Could you check a few things on this model? Use its own coordinates, in mm. A direction names the side the tool comes from. Coordinates: 2 decimals unless noted, no trailing zeros. Order: outer loops, then holes, each group sorted by start corner. A loop starts at its lowest first (then second) coordinate and runs counter-clockwise, first axis right, second up. Notation, with made-up numbers: (-4, 12) -> (42, 12) arc R23 cw to (42, 21) -> close; hole circle Ø3 at (-13.75, -23). An arc over 180 degrees is marked (long way). Put each result on its own line as item: value. Start each with the question number.
Q1. Will these pins go through, and if not, where does the flat tip stop? pin 1 (2.5 mm diameter, centred on x = 137, z = 3.5, fed in from -Y); pin 2 (1.5 mm diameter, centred on y = 76.5, z = 3.5, fed in from +X); pin 3 (2.5 mm diameter, centred on y = 18, z = 2, fed in from -X).
Q2. If we section it at B-B (y = 36): Please give me the cut outline in (x, z).
Q3. We'd pull the mould along X, two halves only. Please class faces 4 (the face through (123, 45, 4.762)), 5 (the face through (187.07, 91.19, 2.35)), 6 (the face through (29.374, 100.071, 2.348)): +X half, -X half, draft (parallel to the pull), parting line (faces both ways), or undercut.
Q4. For faces 1 (the face through (112.438, -12.344, 2.348)), 2 (the face through (186.33, 19, 2)), 3 (the face through (21.23, 20, 2)), which set-ups out of +Z, -Z, +X, -X, +Y, -Y let a thin tool reach every point of the face, with its end or its side?
Q5. If we section it at A-A (x = 133): Please give me the cut outline in (y, z), and give its area (3 significant figures).
Q6. Please list where these lines run through material, in increasing order: line 1 along X through (y, z) = (99, 3); line 2 along X through (y, z) = (45.5, 4.15); line 3 along Y through (x, z) = (34, 4.35).
Q7. If we section it at C-C (z = 2.65): Count the separate pieces of the cut face and the enclosed holes in it, and give its area (3 significant figures).
from build123d import *

# Parameters (mm, degrees)
BOSS_EXTRUDE1_DEPTH  = 4.7625
M4_CLEARANCE_HOLE1_D = 4.5


with BuildPart() as part:
    # Sketch2 → Boss-Extrude1 (new body)
    with BuildSketch(Plane.XY):
        with BuildLine():
            Line((183.553261784, 104.332754576), (181.480626284, 102.260119075))
            ThreePointArc((181.480626284, 102.260119075), (178.236392795, 100.092391562), (174.409558472, 99.331186887))
            Line((174.409558472, 99.331186887), (117.978290457, 99.331186887))
            ThreePointArc((117.978290457, 99.331186887), (112.506161662, 100.961252213), (108.818018348, 105.320025597))
            ThreePointArc((108.818018348, 105.320025597), (103.779868689, 108.613886887), (98.741719029, 105.320025597))
            ThreePointArc((98.741719029, 105.320025597), (95.053575715, 100.961252213), (89.58144692, 99.331186887))
            Line((89.58144692, 99.331186887), (33.150178905, 99.331186887))
            ThreePointArc((33.150178905, 99.331186887), (29.323344582, 100.092391562), (26.079111093, 102.260119075))
            Line((26.079111093, 102.260119075), (24.006475593, 104.332754576))
            ThreePointArc((24.006475593, 104.332754576), (16.228301, 104.332754576), (16.228301, 96.554579982))
            Line((16.228301, 96.554579982), (18.3009365, 94.481944482))
            ThreePointArc((18.3009365, 94.481944482), (20.468664014, 91.237710994), (21.229868689, 87.41087667))
            Line((21.229868689, 87.41087667), (21.229868689, 56.908391119))
            ThreePointArc((21.229868689, 56.908391119), (20.090461192, 54.112499396), (17.321363425, 52.909437667))
            ThreePointArc((17.321363425, 52.909437667), (11.947168689, 47.41087667), (17.321363425, 41.912315673))
            ThreePointArc((17.321363425, 41.912315673), (20.090461192, 40.709253944), (21.229868689, 37.913362221))
            Line((21.229868689, 37.913362221), (21.229868689, 1.251497104))
            ThreePointArc((21.229868689, 1.251497104), (20.468664014, -2.57533722), (18.3009365, -5.819570708))
            Line((18.3009365, -5.819570708), (16.228301, -7.892206209))
            ThreePointArc((16.228301, -7.892206209), (16.228301, -15.670380802), (24.006475593, -15.670380802))
            Line((24.006475593, -15.670380802), (26.079111093, -13.597745301))
            ThreePointArc((26.079111093, -13.597745301), (29.323344582, -11.430017788), (33.150178905, -10.668813113))
            Line((33.150178905, -10.668813113), (89.58144692, -10.668813113))
            ThreePointArc((89.58144692, -10.668813113), (95.053575715, -12.298878439), (98.741719029, -16.657651823))
            ThreePointArc((98.741719029, -16.657651823), (103.779868689, -19.951513113), (108.818018348, -16.657651823))
            ThreePointArc((108.818018348, -16.657651823), (112.506161662, -12.298878439), (117.978290457, -10.668813113))
            Line((117.978290457, -10.668813113), (174.409558472, -10.668813113))
            ThreePointArc((174.409558472, -10.668813113), (178.236392795, -11.430017788), (181.480626284, -13.597745301))
            Line((181.480626284, -13.597745301), (183.553261784, -15.670380802))
            ThreePointArc((183.553261784, -15.670380802), (191.331436377, -15.670380802), (191.331436377, -7.892206209))
            Line((191.331436377, -7.892206209), (189.258800877, -5.819570708))
            ThreePointArc((189.258800877, -5.819570708), (187.091073363, -2.57533722), (186.329868689, 1.251497104))
            Line((186.329868689, 1.251497104), (186.329868689, 37.913362221))
            ThreePointArc((186.329868689, 37.913362221), (187.469276185, 40.709253944), (190.238373952, 41.912315673))
            ThreePointArc((190.238373952, 41.912315673), (195.612568689, 47.41087667), (190.238373952, 52.909437667))
            ThreePointArc((190.238373952, 52.909437667), (187.469276185, 54.112499396), (186.329868689, 56.908391119))
            Line((186.329868689, 56.908391119), (186.329868689, 87.41087667))
            ThreePointArc((186.329868689, 87.41087667), (187.091073363, 91.237710994), (189.258800877, 94.481944482))
            Line((189.258800877, 94.481944482), (191.331436377, 96.554579982))
            ThreePointArc((191.331436377, 96.554579982), (191.331436377, 104.332754576), (183.553261784, 104.332754576))
        make_face()
    extrude(amount=BOSS_EXTRUDE1_DEPTH)

    # M4 Clearance Hole1 (through all)
    with Locations(Plane.XY.offset(4.7625)):
        with Locations((17.447168689, 47.41087667), (20.117388296, 100.443667279), (103.779868689, 103.113886887), (187.442349081, 100.443667279), (190.112568689, 47.41087667), (187.442349081, -11.781293505), (103.779868689, -14.451513113), (20.117388296, -11.781293505)):
            Hole(M4_CLEARANCE_HOLE1_D / 2)


solid = part.part
The answers:
1. pin 1: y = -10.67
1. pin 2: x = 186.33
1. pin 3: x = 21.23
2. outline: (21.23, 0) -> (186.33, 0) -> (186.33, 4.76) -> (21.23, 4.76) -> close
3. face 4: draft
3. face 5: +X half
3. face 6: undercut
4. face 1: +Z, -Z, -Y
4. face 2: +Z, -Z, +X
4. face 3: +Z, -Z, -X
5. outline: (-10.67, 0) -> (99.33, 0) -> (99.33, 4.76) -> (-10.67, 4.76) -> close
5. area: 524 mm^2
6. line 1: 14.81 to 18.39, 21.84 to 185.72, 189.17 to 192.75
6. line 2: 12.29 to 16.26, 18.64 to 188.92, 191.3 to 195.27
6. line 3: -10.67 to 99.33
7. separate pieces: 1
7. enclosed holes: 8
7. area: 18,900 mm^2
